The listing builds one solid part. Answer for the finished solid, in the listing's coordinates (mm). Face numbers are marked on the shaded views. A direction names the side the tool comes from. Coordinates: 2 decimals unless noted, no trailing zeros. Loops run counter-clockwise (first coordinate to the right, second up) from the corner with the lowest first, then second, coordinate; pieces in that order, holes last. Notation, with made-up numbers: (43.5, -25) - (51.5, -25) arc R22 cw to (51.5, 7) - close; hole circle Ø6 at (-23, -36). An arc over 180 degrees is marked (long way). Return JSON: item names as keys, results as strings. Group by question number.
1. Each of these flat-tipped pins is pushed along its axis until it touches: P1, Ø1, axis at x = -12.5, z = 5, coming from the -Y side; P2, Ø0.7, axis at y = -4, z = 3, coming from the -X side. Where does it stop, or does it pass through?
2. Section B-B (z = 5) is taken. Write down the section's boundary in (x, y) (3 decimals), and give its area (3 significant figures).
3. Which of the six approach directions +Z, -Z, +X, -X, +Y, -Y give full straight-line access (tool end or side, diameter ignored) to the marked faces 1, 2 and 3?
4. Section D-D (z = 8.25) is taken. Write down the section's boundary in (x, y) (3 decimals).
5. Find the intervals of material crossed by line 1 along Y through (x, z) = (-25.25, 7); line 2 along X through (y, z) = (-4.5, 2.75); line 3 along Y through (x, z) = (-20, 0.75), in increasing order.
6. The mould has two halves that part along X. Classify the marked faces 4, 5 and 6: pulls with the +X half, pulls with the -X half, needs draft (parallel to the pull), parting line crosses it, or undercut.
7. Section A-A (x = -23.5) is taken. Write down the section's boundary in (y, z).
8. Section C-C (y = 0.75) is taken. Write down the section's boundary in (x, z).
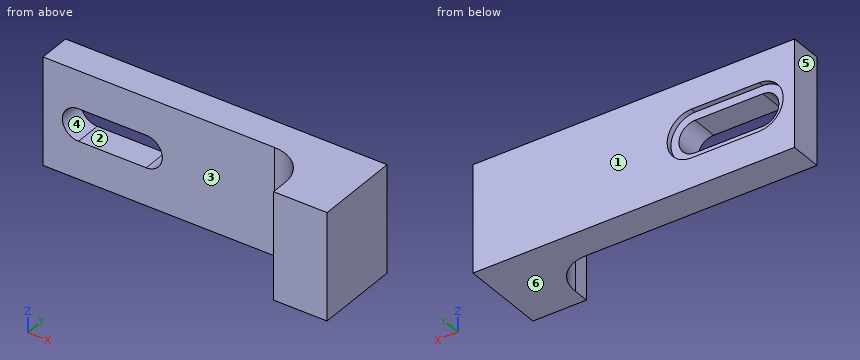
```python
from build123d import *

# Parameters (mm, degrees)
PAD_DEPTH       = 10
POCKET_DEPTH    = 8.001
POCKET001_DEPTH = 0.5


with BuildPart() as part:
    # Sketch → Pad (new body)
    with BuildSketch(Plane.XY):
        with BuildLine():
            Line((-30, 0), (-8.401164, 0))
            ThreePointArc((-5, -3.555465), (-5.94439, -1.054359), (-8.401164, 0))
            Line((-5, -3.555465), (-5, -5))
            Line((-5, -5), (0, -5))
            Line((0, -5), (0, 3))
            Line((0, 3), (-30, 3))
            Line((-30, 3), (-30, 0))
        make_face()
    extrude(amount=PAD_DEPTH)

    # Sketch001 (on DatumPlane) → Pocket (cut, through all)
    with BuildSketch(Plane(origin=(0, 3, 0), x_dir=(-1, 0, 0), z_dir=(0, 1, 0))):
        with BuildLine():
            ThreePointArc((20.368423, 6.5), (18.868423, 5), (20.368423, 3.5))
            Line((20.368423, 3.5), (26.690333, 3.5))
            ThreePointArc((26.690333, 3.5), (28.190333, 5), (26.690333, 6.5))
            Line((20.368423, 6.5), (26.690333, 6.5))
        make_face()
    extrude(amount=-POCKET_DEPTH, mode=Mode.SUBTRACT)

    # Sketch002 (on DatumPlane) → Pocket001 (cut)
    with BuildSketch(Plane(origin=(0, 3, 0), x_dir=(-1, 0, 0), z_dir=(0, 1, 0))):
        with BuildLine():
            ThreePointArc((20.368423, 7.249783), (18.118423, 4.999783), (20.368423, 2.749783))
            Line((20.368423, 2.749783), (26.690333, 2.749783))
            ThreePointArc((26.690333, 2.749783), (28.940333, 4.999783), (26.690333, 7.249783))
            Line((20.368423, 7.249783), (26.690333, 7.249783))
        make_face()
    extrude(amount=-POCKET001_DEPTH, mode=Mode.SUBTRACT)


solid = part.part
```
The answers:
{
 "1": {"P1": "stops at y = 0", "P2": "stops at x = -5"},
 "2": {"outline": "(-30, 0) - (-28.19, 0) - (-28.19, 2.5) - (-28.94, 2.5) - (-28.94, 3) - (-30, 3) - close; (-18.868, 0) - (-8.401, 0) arc R3.415 cw to (-5, -3.555) - (-5, -5) - (0, -5) - (0, 3) - (-18.118, 3) - (-18.118, 2.5) - (-18.868, 2.5) - close", "area": "88.8 mm2"},
 "3": {"face 1": "+Z, -Z, +X, -X, +Y", "face 2": "+Y, -Y", "face 3": "+Z, -Z, -X, -Y"},
 "4": {"outline": "(-30, 0) - (-8.401, 0) arc R3.415 cw to (-5, -3.555) - (-5, -5) - (0, -5) - (0, 3) - (-30, 3) - close"},
 "5": {"line 1": "y = 0 to 2.5", "line 2": "x = -5 to 0", "line 3": "y = 0 to 3"},
 "6": {"face 4": "undercut", "face 5": "pulls with the -X half", "face 6": "needs draft"},
 "7": {"outline": "(0, 0) - (3, 0) - (3, 2.75) - (2.5, 2.75) - (2.5, 3.5) - (0, 3.5) - close; (0, 6.5) - (2.5, 6.5) - (2.5, 7.25) - (3, 7.25) - (3, 10) - (0, 10) - close"},
 "8": {"outline": "(-30, 0) - (0, 0) - (0, 10) - (-30, 10) - close; hole (-26.69, 3.5) - (-20.37, 3.5) arc R1.5 ccw to (-20.37, 6.5) - (-26.69, 6.5) arc R1.5 ccw to start"}
}
